Here's how the part is built. I have some questions about the finished solid (model axes, mm). A direction names the side the tool comes from. Round coordinates to 2 decimals unless told otherwise and drop trailing zeros. Order: outer loops, then holes, each group sorted by start corner. A loop starts at its lowest first (then second) coordinate and runs counter-clockwise, first axis right, second up. Notation, with made-up numbers: (-25, -31) - (18, -31) arc R23 ccw to (18, -2) - close; hole circle Ø9 at (28, 16.25). An arc over 180 degrees is marked (long way). Answer as a JSON object with one key per item and string values.
```python
from build123d import *

# Parameters (mm, degrees)
SKETCH_8_R      = 14.5
SKETCH_8_R_2    = 10
EXTRUDE_1_DEPTH = 31
SKETCH_10_R     = 23.5
SKETCH_10_R_2   = 14.5
EXTRUDE_2_DEPTH = 17
EXTRUDE_START   = -5
SKETCH_11_R     = 31
SKETCH_11_R_2   = 23.5
EXTRUDE_3_DEPTH = 25
SKETCH_13_W     = 41
SKETCH_13_H     = 38
EXTRUDE_4_DEPTH = 14
FILLET_1_R      = 8
FILLET_2_R      = 5
FILLET_3_R      = 5
FILLET_4_R      = 8
FILLET_5_R      = 1
FILLET_6_R      = 1


with BuildPart() as part:
    # Эскиз8 → Вытянуть1 (new body)
    with BuildSketch(Plane.XY):
        with Locations((50, -1.5)):
            Circle(SKETCH_8_R)
        with Locations((50, -1.5)):
            Circle(SKETCH_8_R_2, mode=Mode.SUBTRACT)
    extrude(amount=EXTRUDE_1_DEPTH)

    # Эскиз10 → Вытянуть2 (add)
    with BuildSketch(Plane.XY.offset(10)):
        with Locations((50, -1.5)):
            Circle(SKETCH_10_R)
        with Locations((50, -1.5)):
            Circle(SKETCH_10_R_2, mode=Mode.SUBTRACT)
    extrude(amount=EXTRUDE_2_DEPTH)

    # Эскиз11 → Вытянуть3 (add)
    with BuildSketch(Plane.XY.offset(10).offset(EXTRUDE_START)):
        with Locations((50, -1.5)):
            Circle(SKETCH_11_R)
        with Locations((50, -1.5)):
            Circle(SKETCH_11_R_2, mode=Mode.SUBTRACT)
    extrude(amount=EXTRUDE_3_DEPTH)

    # Эскиз13 → Вытянуть4 (add)
    # profile 1 of 2: a face of its own
    with BuildSketch(Plane(origin=(0, -36, 0), x_dir=(-1, 0, 0), z_dir=(0, 1, 0))):
        with Locations((-7.5, 17.5)):
            Rectangle(SKETCH_13_W, SKETCH_13_H)
        with BuildLine():
            Line((-4.740103958, 23.994802079), (0, 24))
            ThreePointArc((0, 24), (6.5, 17.5), (0, 11))
            Line((0, 11), (-5, 11))
            ThreePointArc((-5, 11), (-11.49870039, 17.629974008), (-4.740103958, 23.994802079))
        make_face(mode=Mode.SUBTRACT)
    # profile 2 of 2: a face of its own
    with BuildSketch(Plane(origin=(0, -36, 0), x_dir=(-1, 0, 0), z_dir=(0, 1, 0))):
        with Locations((-92.5, 17.5)):
            Rectangle(SKETCH_13_W, SKETCH_13_H)
        with BuildLine():
            Line((-95, 11), (-100, 11))
            ThreePointArc((-100, 11), (-106.5, 17.5), (-100, 24))
            Line((-100, 24), (-95.259896042, 23.994802079))
            ThreePointArc((-95.259896042, 23.994802079), (-88.50129961, 17.629974008), (-95, 11))
        make_face(mode=Mode.SUBTRACT)
    extrude(amount=EXTRUDE_4_DEPTH)

    # Скругление1
    fillet_1_edges = [part.edges().sort_by_distance(p)[0] for p in [
        (26.745968092, -22, 17.5),
    ]]
    fillet(fillet_1_edges, radius=FILLET_1_R)

    # Скругление2
    fillet_2_edges = [part.edges().sort_by_distance(p)[0] for p in [
        (28, -23.340329668, 17.5),
    ]]
    fillet(fillet_2_edges, radius=FILLET_2_R)

    # Скругление3
    fillet_3_edges = [part.edges().sort_by_distance(p)[0] for p in [
        (72, -23.340329668, 17.5),
    ]]
    fillet(fillet_3_edges, radius=FILLET_3_R)

    # Скругление4
    fillet_4_edges = [part.edges().sort_by_distance(p)[0] for p in [
        (73.254031908, -22, 17.5),
    ]]
    fillet(fillet_4_edges, radius=FILLET_4_R)

    # Скругление5
    fillet_5_edges = [part.edges().sort_by_distance(p)[0] for p in [
        (28, -29, 36.5),
        (28, -29, -1.5),
        (72, -29, -1.5),
        (72, -29, 36.5),
    ]]
    fillet(fillet_5_edges, radius=FILLET_5_R)

    # Скругление6
    fillet_6_edges = [part.edges().sort_by_distance(p)[0] for p in [
        (-13, -29, -1.5),
        (-13, -29, 36.5),
        (113, -29, 36.5),
        (113, -29, -1.5),
    ]]
    fillet(fillet_6_edges, radius=FILLET_6_R)


solid = part.part
```
1. If I drill on L1, parallel to Y at x = 50, z = 27.75; L2, parallel to X at y = -1, z = 7; L3, parallel to X at y = -2, z = 15, over which ranges is the centre line in solid material (lowest first)? Write a range as [from, to].
Responses:
{"L1": "[-32.5, -25], [-16, -11.5], [8.5, 13], [22, 29.5]", "L2": "[19, 26.51], [35.51, 40.01], [59.99, 64.49], [73.49, 81]", "L3": "[19, 40.01], [59.99, 81]"}
2. For faces 5 (the face through (106.5, -29.1, 17.4)), 6 (the face through (39, -12, 10)), 7 (the face through (39, -12, 27)), which set-ups out of +Z, -Z, +X, -X, +Y, -Y let a thin tool reach every point of the face, with its end or its side?
Responses:
{"face 5": "+Y, -Y", "face 6": "-Z", "face 7": "+Z"}
3. Thinking about a two-plate mould opening in Y: for faces 1 (the face through (53, 8.4, 31)), 2 (the face through (50.82, 29.49, 17.32)), 3 (the face through (49.8, -32.5, 17.3)), 4 (the face through (97, -22, 26)), which applies, pulls with the +Y half, pulls with the -Y half, needs draft (parallel to the pull), parting line crosses it, or undercut?
Responses:
{"face 1": "needs draft", "face 2": "undercut", "face 3": "pulls with the -Y half", "face 4": "pulls with the +Y half"}
4. Imagine slicing it at C-C (z = 17.5). List the corners of the cut face in (x, y) for me, plus the area to 3 significant figures.
Responses:
{"outline": "(-13, -36) - (-6.5, -36) - (-6.5, -22) - (-13, -22) - close; (11.5, -36) - (28, -36) - (28, -33.23) arc R5 cw to (35.36, -28.83) arc R31 ccw to (64.64, -28.83) arc R5 cw to (72, -33.23) - (72, -36) - (88.5, -36) - (88.5, -22) - (86.94, -22) arc R8 cw to (79.36, -11.44) arc R31 ccw (long way) to (20.64, -11.44) arc R8 cw to (13.06, -22) - (11.5, -22) - close; (106.5, -36) - (113, -36) - (113, -22) - (106.5, -22) - close; hole circle Ø20 at (50, -1.5)", "area": "3,460 mm2"}
5. Imagine slicing it at B-B (y = -1.5). List the corners of the cut face in (x, z) for me.
Responses:
{"outline": "(19, 5) - (26.5, 5) - (26.5, 10) - (35.5, 10) - (35.5, 0) - (40, 0) - (40, 31) - (35.5, 31) - (35.5, 27) - (26.5, 27) - (26.5, 30) - (19, 30) - close; (60, 0) - (64.5, 0) - (64.5, 10) - (73.5, 10) - (73.5, 5) - (81, 5) - (81, 30) - (73.5, 30) - (73.5, 27) - (64.5, 27) - (64.5, 31) - (60, 31) - close"}
6. For P1, Ø4, axis at y = 3, z = 24, coming from the -X side; P2, Ø23, axis at x = 50, y = 1.5, coming from the +Z side; P3, Ø14.5, axis at x = 49, y = 2.5, coming from the -Z side, each with a flat end and sliding along its axis, tell me the tip position at first contact or that it passes through.
Responses:
{"P1": "x = 19.1", "P2": "z = 31", "P3": "z = 0"}
7. Imagine slicing it at D-D (x = 68). List the corners of the cut face in (y, z) for me, plus the area to 3 significant figures.
Responses:
{"outline": "(-28.33, 5) - (-16.61, 5) - (-16.61, 10) - (13.61, 10) - (13.61, 5) - (23.74, 5) - (23.74, 30) - (13.61, 30) - (13.61, 27) - (-16.61, 27) - (-16.61, 30) - (-28.33, 30) - close", "area": "1,060 mm2"}
8. Imagine slicing it at A-A (x = 50). List the corners of the cut face in (y, z) for me, plus the area to 3 significant figures.
Responses:
{"outline": "(-32.5, 5) - (-25, 5) - (-25, 10) - (-16, 10) - (-16, 0) - (-11.5, 0) - (-11.5, 31) - (-16, 31) - (-16, 27) - (-25, 27) - (-25, 30) - (-32.5, 30) - close; (8.5, 0) - (13, 0) - (13, 10) - (22, 10) - (22, 5) - (29.5, 5) - (29.5, 30) - (22, 30) - (22, 27) - (13, 27) - (13, 31) - (8.5, 31) - close", "area": "960 mm2"}
